Could you check a few things on this model? Use its own coordinates, in mm. A direction names the side the tool comes from. Round coordinates to 2 decimals unless told otherwise and drop trailing zeros. Loops run counter-clockwise (first coordinate to the right, second up) from the corner with the lowest first, then second, coordinate; pieces in that order, holes last. Notation, with made-up numbers: M 86,-29 L 135,-29 A25 cw 135,-13 Z; hole C -12,-10 d10. An arc over 180 degrees is marked long. Answer in a Markdown table with one row per item.
```python
from build123d import *

# Parameters (mm, degrees)
F0_W     = 228.6
F0_H     = 152.4
F1_DEPTH = 76.2
F2_W     = 76.2
F2_H     = 127
F3_DEPTH = 76.2
F4_R     = 25.4
F5_W     = 50.8
F5_H     = 50.8
F6_DEPTH = 25.4


with BuildPart() as f1:
    # F0 (on Right) → F1 (new body, symmetric)
    with BuildSketch(Plane.YZ):
        with Locations((-114.3, 76.2)):
            Rectangle(F0_W, F0_H)
    extrude(amount=F1_DEPTH, both=True)

    # F2 (on face) → F3 (cut)
    with BuildSketch(Plane(origin=(-76.2, 0, 0), x_dir=(0, -1, 0), z_dir=(-1, 0, 0))):
        with Locations((114.3, 88.9)):
            Rectangle(F2_W, F2_H)
    extrude(amount=-F3_DEPTH, mode=Mode.SUBTRACT)

    # F4
    f4_edges = [f1.edges().sort_by_distance(p)[0] for p in [
        (76.2, -228.6, 76.2),
    ]]
    fillet(f4_edges, radius=F4_R)

    # F5 (on face) → F6 (cut)
    with BuildSketch(Plane.XZ.offset(228.6)):
        with Locations((0, 76.2)):
            Rectangle(F5_W, F5_H)
    extrude(amount=-F6_DEPTH, mode=Mode.SUBTRACT)


solid = f1.part
```
1) I need wall thicknesses on line 1 (Y direction, x = -66, z = 85); line 2 (Z direction, x = -20.5, y = -211.5); line 3 (X direction, y = -142, z = 68). Which ranges of each line are inside material? Lowest first, please.
Computed:
| item | result |
|---|---|
| line 1 | y = -228.6 to -152.4, -76.2 to 0 |
| line 2 | z = 0 to 50.8, 101.6 to 152.4 |
| line 3 | x = 0 to 76.2 |
2) I want a section at C-C, the plane y = -206. Please give me the cut outline in (x, z).
Computed:
| item | result |
|---|---|
| outline | M -76.2,0 L 76.05,0 L 76.05,152.4 L -76.2,152.4 Z; hole M -25.4,50.8 L 25.4,50.8 L 25.4,101.6 L -25.4,101.6 Z |
3) I want a section at D-D, the plane z = 70.5. Please give me the cut outline in (x, y), plus the area to 3 significant figures.
Computed:
| item | result |
|---|---|
| outline | M -76.2,-228.6 L -25.4,-228.6 L -25.4,-203.2 L 25.4,-203.2 L 25.4,-228.6 L 50.8,-228.6 A25.4 ccw 76.2,-203.2 L 76.2,0 L -76.2,0 L -76.2,-76.2 L 0,-76.2 L 0,-152.4 L -76.2,-152.4 Z |
| area | 27,600 mm² |
4) Will these pins go through, and if not, where does the flat tip stop? P1, Ø15, axis at x = 7, z = 82.5, coming from the -Y side; P2, Ø12, axis at x = 45.5, z = 62, coming from the +Y side; P3, Ø12.5, axis at y = -214, z = 70.5, coming from the +X side; P4, Ø23, axis at y = -115.5, z = 61.5, coming from the -X side.
Computed:
| item | result |
|---|---|
| P1 | stops at y = -203.2 |
| P2 | stops at y = 0 |
| P3 | stops at x = 75.79 |
| P4 | stops at x = 0 |
5) Which directions (+Z, -Z, +X, -X, +Y, -Y) give clear straight access to the entire face, cutting with the end or side of a thin tool? Please do faces 5 (the face through (-76.2, -65, 77)), 6 (the face through (0, -216, 50.8)), 7 (the face through (-39, -76.2, 88)).
Computed:
| item | result |
|---|---|
| face 5 | +Z, -Z, -X, +Y, -Y |
| face 6 | -Y |
| face 7 | +Z, -X |
6) If we mould it in two halves opening along Z, with no side actions, what happens to faces 1 (the face through (25.4, -216, 76)), 2 (the face through (1, -116, 152.4)), 3 (the face through (0, -203.2, 77)), 4 (the face through (0, -114, 90))? For each: released by +Z, released by -Z, zero draft, split by the parting line, or undercut.
Computed:
| item | result |
|---|---|
| face 1 | undercut |
| face 2 | released by +Z |
| face 3 | undercut |
| face 4 | zero draft |
7) I want a section at A-A, the plane x = 15.5. Please give me the cut outline in (y, z), plus the area to 3 significant figures.
Computed:
| item | result |
|---|---|
| outline | M -228.6,0 L 0,0 L 0,152.4 L -228.6,152.4 L -228.6,101.6 L -203.2,101.6 L -203.2,50.8 L -228.6,50.8 Z |
| area | 33,500 mm² |
8) I want a section at B-B, the plane z = 35. Please give me the cut outline in (x, y), plus the area to 3 significant figures.
Computed:
| item | result |
|---|---|
| outline | M -76.2,-228.6 L 50.8,-228.6 A25.4 ccw 76.2,-203.2 L 76.2,0 L -76.2,0 L -76.2,-76.2 L 0,-76.2 L 0,-152.4 L -76.2,-152.4 Z |
| area | 28,900 mm² |
